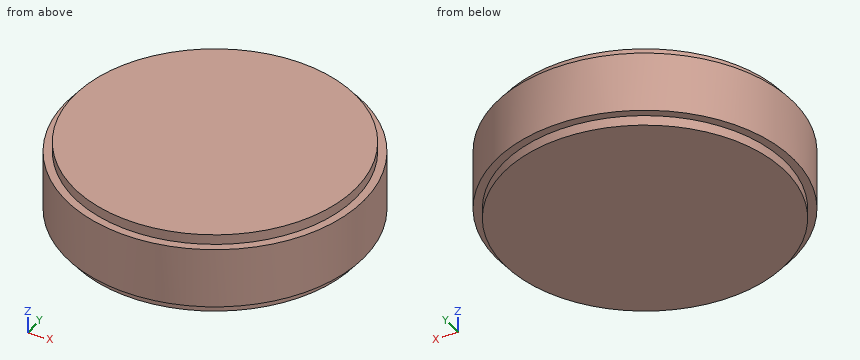
from build123d import *

# Parameters (mm, degrees)
SKETCH1_R           = 74
BOSS_EXTRUDE1_DEPTH = 20
SKETCH2_R           = 74
SKETCH2_R_2         = 70
CUT_EXTRUDE1_DEPTH  = 5
CUT_EXTRUDE2_START  = -5
SKETCH3_R           = 74
SKETCH3_R_2         = 70
CUT_EXTRUDE2_DEPTH  = 5


with BuildPart() as part:
    # Sketch1 → Boss-Extrude1 (new, symmetric)
    with BuildSketch(Plane.XY):
        Circle(SKETCH1_R)
    extrude(amount=BOSS_EXTRUDE1_DEPTH, both=True)

    # Sketch2 → Cut-Extrude1 (cut)
    with BuildSketch(Plane.XY.offset(20)):
        Circle(SKETCH2_R)
        Circle(SKETCH2_R_2, mode=Mode.SUBTRACT)
    extrude(amount=-CUT_EXTRUDE1_DEPTH, mode=Mode.SUBTRACT)

    # Sketch3 → Cut-Extrude2 (cut)
    with BuildSketch(Plane(origin=(0, 0, -20), x_dir=(-1, 0, 0), z_dir=(0, 0, -1)).offset(CUT_EXTRUDE2_START)):
        Circle(SKETCH3_R)
        with Locations(Location((0, 0, 0), (0, 0, 180))):
            Circle(SKETCH3_R_2, mode=Mode.SUBTRACT)
    extrude(amount=CUT_EXTRUDE2_DEPTH, mode=Mode.SUBTRACT)


solid = part.part
Geometry check sheet. Reference: the model listing, model coordinates, mm. Round coordinates to 2 decimals unless told otherwise and drop trailing zeros. Order: outer loops, then holes, each group sorted by start corner. A loop starts at its lowest first (then second) coordinate and runs counter-clockwise, first axis right, second up. Notation, with made-up numbers: (84.5, 13.25) - (128.5, 13.25) arc R12 cw to (128.5, 22.25) - close; hole circle Ø8 at (2, -34). An arc over 180 degrees is marked (long way). One line per question, with ' | ' between items. Start each with the question number.
(1) Depth check by flat-ended pin: pin 1 Ø12 at (x, z) = (-39.5, -8.5) entering from -Y; pin 2 Ø3 at (x, z) = (53.5, -1.5) entering from -Y; pin 3 Ø1.5 at (y, z) = (37.5, 10.5) entering from -X. Enter the tip coordinate at first touch or a pass-through.
(2) Sectioned sample at A-A on x = -22.5. Record the cut outline in (y, z).
(3) Sectioned sample at C-C on z = -8.5. Record the cut outline in (x, y).
(4) Sectioned sample at B-B on y = -61.5. Record the cut outline in (x, z).
(5) Thickness scan on L1, parallel to Z at x = -49.5, y = 51.5; L2, parallel to X at y = 38, z = 5.5; L3, parallel to Y at x = 2.5, z = 13. Record the ranges inside material, lowest first. Write a range as [from, to].
Conclusion:
1) pin 1: stops at y = -65.98 | pin 2: stops at y = -52.65 | pin 3: stops at x = -64.23
2) outline: (-70.5, -15) - (-66.29, -15) - (-66.29, -20) - (66.29, -20) - (66.29, -15) - (70.5, -15) - (70.5, 15) - (66.29, 15) - (66.29, 20) - (-66.29, 20) - (-66.29, 15) - (-70.5, 15) - close
3) outline: circle Ø148 at (0, 0)
4) outline: (-41.16, -15) - (-33.43, -15) - (-33.43, -20) - (33.43, -20) - (33.43, -15) - (41.16, -15) - (41.16, 15) - (33.43, 15) - (33.43, 20) - (-33.43, 20) - (-33.43, 15) - (-41.16, 15) - close
5) L1: z = [-15, 15] | L2: x = [-63.5, 63.5] | L3: y = [-73.96, 73.96]
